from build123d import *

# Parameters (mm, degrees)
EXTRUDE_1_DEPTH     = 5
FILLET_2_R          = 1
HOLE_WIZARD_M3_1_D  = 2.5
SKETCH_5_R          = 5
CUT_EXTRUDE_1_DEPTH = 5
HOLE_WIZARD_M5_1_D  = 4.2
SKETCH_7_R          = 10
CUT_EXTRUDE_2_DEPTH = 80.366239674


with BuildPart() as part:
    # 草图1 → 凸台-拉伸1 (new body)
    with BuildSketch(Plane.XY):
        Polygon((-57, 35), (-57, -35), (-12, -35), (-12, -55), (12, -55), (12, -35), (57, -35), (57, 35), (12, 35), (12, 55), (-12, 55), (-12, 35), align=None)
    extrude(amount=EXTRUDE_1_DEPTH)

    # 圆角2
    fillet_2_edges = [part.edges().sort_by_distance(p)[0] for p in [
        (-12, 55, 2.5),
        (12, 55, 2.5),
        (57, 35, 2.5),
        (57, -35, 2.5),
        (12, -55, 2.5),
        (-12, -55, 2.5),
        (-57, -35, 2.5),
        (-57, 35, 2.5),
    ]]
    fillet(fillet_2_edges, radius=FILLET_2_R)

    # M3 螺纹孔的螺纹孔钻头1 (through all)
    with Locations(Plane(origin=(-23, 9, 5), x_dir=(1, 0, 0), z_dir=(0, 0, 1))):
        with Locations((0, 0), (0, -18)):
            hole_wizard_m3_1 = Hole(HOLE_WIZARD_M3_1_D / 2)

    # 镜向1: M3 螺纹孔的螺纹孔钻头1 across plane
    add(hole_wizard_m3_1.mirror(Plane(origin=(0, 0, 0), x_dir=(0, 0, 1), z_dir=(1, 0, 0))), mode=Mode.SUBTRACT)

    # 草图5 → 切除-拉伸1 (cut)
    with BuildSketch(Plane.XY.offset(5)):
        with Locations((-48, 26)):
            Circle(SKETCH_5_R)
        with Locations((-48, -26)):
            Circle(SKETCH_5_R)
    cut_extrude_1 = extrude(amount=-CUT_EXTRUDE_1_DEPTH, mode=Mode.SUBTRACT)

    # 镜向2: 切除-拉伸1 across plane
    add(cut_extrude_1.mirror(Plane(origin=(0, 0, 0), x_dir=(0, 0, 1), z_dir=(1, 0, 0))), mode=Mode.SUBTRACT)

    # M5 螺纹孔的螺纹孔钻头1 (through all)
    with Locations(Plane(origin=(0, 47.5, 5), x_dir=(1, 0, 0), z_dir=(0, 0, 1))):
        with Locations((0, 0)):
            hole_wizard_m5_1 = Hole(HOLE_WIZARD_M5_1_D / 2)

    # 镜向3: M5 螺纹孔的螺纹孔钻头1 across plane
    add(hole_wizard_m5_1.mirror(Plane.ZX), mode=Mode.SUBTRACT)

    # 草图7 → 切除-拉伸2 (cut, through all)
    with BuildSketch(Plane.XY.offset(5)):
        with Locations((0, 9)):
            Circle(SKETCH_7_R)
    extrude(amount=-CUT_EXTRUDE_2_DEPTH, mode=Mode.SUBTRACT)


solid = part.part
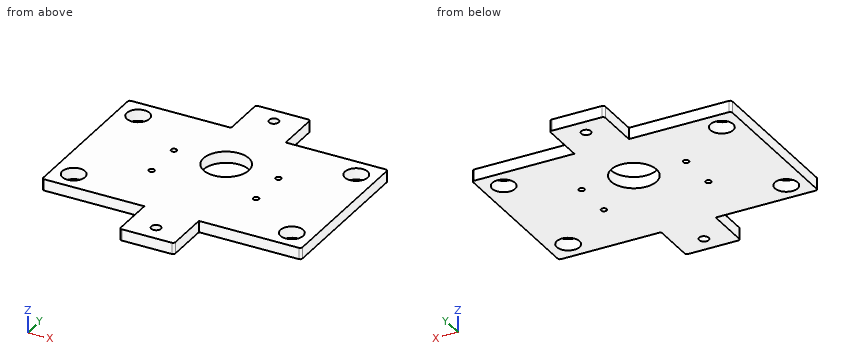
Design review of the part built by this model. Coordinates are the model's own, in mm. Give positions to 0.01 mm unless a question says otherwise; leave off trailing zeros. Write each loop counter-clockwise with the first axis right and the second up, starting at its lowest first coordinate (ties: lowest second). Pieces come first, ordered by that corner, then holes. Notation, with made-up numbers: M 74.5,44.25 L 114.5,44.25 A26 ccw 114.5,59.25 Z; hole C 79.5,-32 d10. An arc over 180 degrees is marked long. Return JSON: item names as keys, results as strings. Group by question number.
Item 1: Clearance check with flat-ended pins moving along their axes: pin 1 Ø13 at (x, y) = (48, 26) entering from -Z; pin 2 Ø2.5 at (x, z) = (-40.5, 3.5) entering from -Y. State where each tip first meets the part, or that it passes through.
Item 2: Take a section at C-C (z = 1.75). Count the separate pieces of the cut face and the enclosed holes in it, plus the area to 3 significant figures.
Item 3: Take a section at D-D (y = -47.5). Give the boundary of the cut face in (x, z), plus the area to 3 significant figures.
Item 4: Take a section at A-A (y = 26). Give the boundary of the cut face in (x, z).
Item 5: Wall thickness on line 1 along Y through (x, z) = (23, 3.6); line 2 along Y through (x, z) = (48, 3.45); line 3 along Y through (x, z) = (0, 3.65): over which ranges is each line inside the solid? List them lowest first.
Item 6: Take a section at B-B (x = -48). Give the boundary of the cut face in (y, z).
Return value:
{
 "1": {"pin 1": "stops at z = 0", "pin 2": "stops at y = -35"},
 "2": {"separate pieces": "1", "enclosed holes": "11", "area": "8,260 mm2"},
 "3": {"outline": "M -12,0 L -2.1,0 L -2.1,5 L -12,5 Z; M 2.1,0 L 12,0 L 12,5 L 2.1,5 Z", "area": "99.0 mm2"},
 "4": {"outline": "M -57,0 L -53,0 L -53,5 L -57,5 Z; M -43,0 L 43,0 L 43,5 L -43,5 Z; M 53,0 L 57,0 L 57,5 L 53,5 Z"},
 "5": {"line 1": "y = -35 to -10.25, -7.75 to 7.75, 10.25 to 35", "line 2": "y = -35 to -31, -21 to 21, 31 to 35", "line 3": "y = -55 to -49.6, -45.4 to -1, 19 to 45.4, 49.6 to 55"},
 "6": {"outline": "M -35,0 L -31,0 L -31,5 L -35,5 Z; M -21,0 L 21,0 L 21,5 L -21,5 Z; M 31,0 L 35,0 L 35,5 L 31,5 Z"}
}
